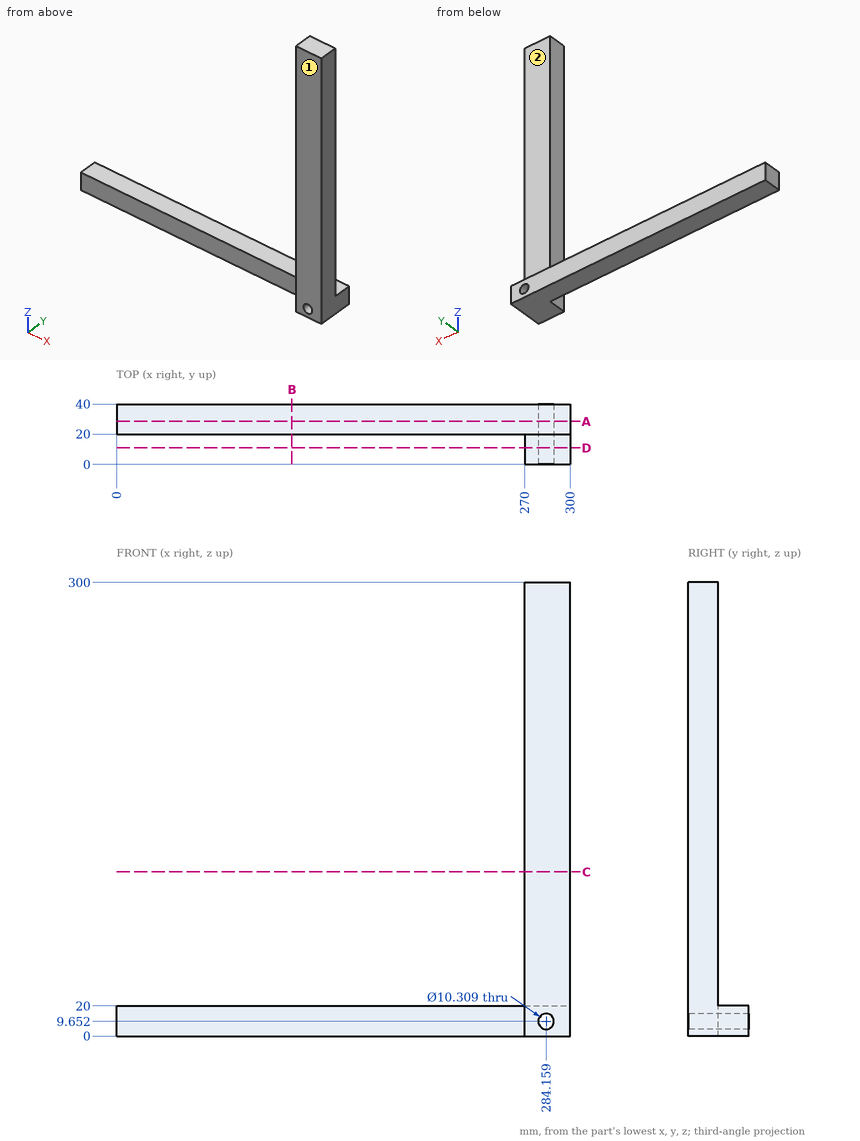
Design review of the part shown in the three views and the two pictorial views. Dimensions are in mm from the part's minimum x, y and z. A direction names the side the tool comes from. Give positions to 0.01 mm unless a question says otherwise; leave off trailing zeros. Write each loop counter-clockwise with the first axis right and the second up, starting at its lowest first coordinate (ties: lowest second). Pieces come first, ordered by that corner, then holes. Notation, with made-up numbers: M 77.5,11 L 98.5,11 A18 cw 98.5,42 Z; hole C 14.5,-25.5 d8. An arc over 180 degrees is marked long. Return JSON: item names as keys, results as strings. Group by question number.
Item 1: Take a section at D-D (y = 11). Give the boundary of the cut face in (x, z) (1 decimal).
Item 2: Clearance check with flat-ended pins moving along their axes: pin 1 Ø16 at (x, y) = (170, 26) entering from +Z; pin 2 Ø16 at (y, z) = (13.5, 89.5) entering from -X; pin 3 Ø6 at (x, z) = (139.5, 10.5) entering from -Y. State where each tip first meets the part, or that it passes through.
Item 3: Take a section at C-C (z = 108.5). Give the boundary of the cut face in (x, y), plus the area to 3 significant figures.
Item 4: Take a section at A-A (y = 28.5). Give the boundary of the cut face in (x, z) (1 decimal), plus the area to 3 significant figures.
Item 5: Tool access review of the marked faces 1 and 2: name each direction out of +Z, -Z, +X, -X, +Y, -Y from which nothing blocks a thin tool from reaching the whole face with its end or side.
Item 6: Wall thickness on line 1 along Z through (x, y) = (33.5, 25); line 2 along X through (y, z) = (5, 49): over which ranges is each line inside the solid? List them lowest first.
Item 7: Take a section at B-B (x = 116). Give the boundary of the cut face in (y, z), plus the area to 3 significant figures.
Return value:
{
 "1": {"outline": "M 270,0 L 300,0 L 300,300 L 270,300 Z; hole C 284.2,9.7 d10.3"},
 "2": {"pin 1": "stops at z = 20", "pin 2": "stops at x = 270", "pin 3": "stops at y = 20"},
 "3": {"outline": "M 270,0 L 300,0 L 300,20 L 270,20 Z", "area": "600 mm2"},
 "4": {"outline": "M 0,0 L 300,0 L 300,20 L 0,20 Z; hole C 284.2,9.7 d10.3", "area": "5,920 mm2"},
 "5": {"face 1": "+Z, -Z, +X, -X, -Y", "face 2": "+Z, +X, -X, +Y"},
 "6": {"line 1": "z = 0 to 20", "line 2": "x = 270 to 300"},
 "7": {"outline": "M 20,0 L 40,0 L 40,20 L 20,20 Z", "area": "400 mm2"}
}
